Geometry check sheet. Reference: the model listing, model coordinates, mm. A direction names the side the tool comes from. Round coordinates to 2 decimals unless told otherwise and drop trailing zeros. Loops run counter-clockwise (first coordinate to the right, second up) from the corner with the lowest first, then second, coordinate; pieces in that order, holes last.
```python
from build123d import *

# Parameters (mm, degrees)
SKETCH1_W               = 30
SKETCH1_H               = 38
BOSS_EXTRUDE1_DEPTH     = 3.175
SKETCH2_W               = 30
SKETCH2_H               = 3.175
BOSS_EXTRUDE2_DEPTH     = 34.825
SKETCH3_R               = 4
CUT_EXTRUDE1_DEPTH      = 60.638751035
SKETCH4_R               = 4
CUT_EXTRUDE2_DEPTH      = 58.667679423
CROQUIS4_R              = 4
CROQUIS4_R_2            = 3.5
SALIENTE_EXTRUIR2_DEPTH = 5
CROQUIS5_W              = 3.979032683
CROQUIS5_H              = 10.100326852
CORTAR_EXTRUIR1_DEPTH   = 36
CROQUIS6_W              = 38
CROQUIS6_H              = 3.175
SALIENTE_EXTRUIR3_DEPTH = 30
CROQUIS7_W              = 3.175
CROQUIS7_H              = 34.825
SALIENTE_EXTRUIR4_DEPTH = 30
CROQUIS8_R              = 3.5
CORTAR_EXTRUIR2_DEPTH   = 30
CROQUIS9_W              = 28.045440503
CROQUIS9_H              = 19.668665091
SALIENTE_EXTRUIR5_DEPTH = 9
CROQUIS10_W             = 26.699428358
CROQUIS10_H             = 12.946692093
CORTAR_EXTRUIR3_DEPTH   = 65
CROQUIS11_R             = 3.5
CORTAR_EXTRUIR4_DEPTH   = 65


with BuildPart() as part:
    # Sketch1 → Boss-Extrude1 (new body)
    with BuildSketch(Plane.XY):
        with Locations((15, 19)):
            Rectangle(SKETCH1_W, SKETCH1_H)
    extrude(amount=BOSS_EXTRUDE1_DEPTH)

    # Sketch2 → Boss-Extrude2 (add)
    with BuildSketch(Plane(origin=(0, 0, 0), x_dir=(-1, 0, 0), z_dir=(0, 0, -1))):
        with Locations((-15, 1.5875)):
            Rectangle(SKETCH2_W, SKETCH2_H)
    extrude(amount=BOSS_EXTRUDE2_DEPTH)

    # Sketch3 → Cut-Extrude1 (cut, through all)
    with BuildSketch(Plane(origin=(0, 0, 0), x_dir=(-1, 0, 0), z_dir=(0, 0, -1))):
        with Locations((-15, 28)):
            Circle(SKETCH3_R)
    extrude(amount=-CUT_EXTRUDE1_DEPTH, mode=Mode.SUBTRACT)

    # Sketch4 → Cut-Extrude2 (cut, through all)
    with BuildSketch(Plane(origin=(0, 3.175, 0), x_dir=(1, 0, 0), z_dir=(0, 1, 0))):
        with Locations(Location((15, 24.825, 0), (0, 0, 180))):
            Circle(SKETCH4_R)
    extrude(amount=-CUT_EXTRUDE2_DEPTH, mode=Mode.SUBTRACT)

    # Croquis4 → Saliente-Extruir2 (add)
    with BuildSketch(Plane(origin=(0, 0, 0), x_dir=(-1, 0, 0), z_dir=(0, 0, -1))):
        with Locations((-15, 28)):
            Circle(CROQUIS4_R)
        with Locations((-15, 28)):
            Circle(CROQUIS4_R_2, mode=Mode.SUBTRACT)
    extrude(amount=-SALIENTE_EXTRUIR2_DEPTH)

    # Croquis5 → Cortar-Extruir1 (cut)
    with BuildSketch(Plane.ZY):
        with Locations((5.164516342, 27.585777405)):
            Rectangle(CROQUIS5_W, CROQUIS5_H)
    extrude(amount=-CORTAR_EXTRUIR1_DEPTH, mode=Mode.SUBTRACT)

    # Croquis6 → Saliente-Extruir3 (add)
    with BuildSketch(Plane.ZY):
        with Locations((-15.825, 1.5875)):
            Rectangle(CROQUIS6_W, CROQUIS6_H)
    extrude(amount=SALIENTE_EXTRUIR3_DEPTH)

    # Croquis7 → Saliente-Extruir4 (add)
    with BuildSketch(Plane.ZY):
        with Locations((1.5875, 20.5875)):
            Rectangle(CROQUIS7_W, CROQUIS7_H)
    extrude(amount=SALIENTE_EXTRUIR4_DEPTH)

    # Croquis8 → Cortar-Extruir2 (cut)
    with BuildSketch(Plane(origin=(0, 0, 0), x_dir=(-1, 0, 0), z_dir=(0, 0, -1))):
        with Locations((15, 28)):
            Circle(CROQUIS8_R)
    extrude(amount=-CORTAR_EXTRUIR2_DEPTH, mode=Mode.SUBTRACT)

    # Croquis9 → Saliente-Extruir5 (add)
    with BuildSketch(Plane(origin=(0, 3.175, 0), x_dir=(1, 0, 0), z_dir=(0, 1, 0))):
        with Locations((15.977279749, 24.990667455)):
            Rectangle(CROQUIS9_W, CROQUIS9_H)
    extrude(amount=-SALIENTE_EXTRUIR5_DEPTH)

    # Croquis10 → Cortar-Extruir3 (cut)
    with BuildSketch(Plane.ZY.offset(30)):
        with Locations((-21.475285821, -6.473346047)):
            Rectangle(CROQUIS10_W, CROQUIS10_H)
    extrude(amount=-CORTAR_EXTRUIR3_DEPTH, mode=Mode.SUBTRACT)

    # Croquis11 → Cortar-Extruir4 (cut)
    with BuildSketch(Plane(origin=(0, 3.175, 0), x_dir=(1, 0, 0), z_dir=(0, 1, 0))):
        with Locations(Location((0, 24.825, 0), (0, 0, 180))):
            Circle(CROQUIS11_R)
    extrude(amount=-CORTAR_EXTRUIR4_DEPTH, mode=Mode.SUBTRACT)


solid = part.part
```
1) Sectioned sample at B-B, the plane y = 28. Record the cut outline in (x, z) (3 decimals).
Report:
outline: (-30, 0) - (-18.5, 0) - (-18.5, 3.175) - (-30, 3.175) - close; (-11.5, 0) - (11.5, 0) - (11.5, 3.175) - (-11.5, 3.175) - close; (18.5, 0) - (30, 0) - (30, 3.175) - (18.5, 3.175) - close
2) Access from +Z, -Z, +X, -X, +Y, -Y to the whole of each face (thin tool, end or side, straight path). Record for faces 1 (the face through (0, 20, 0)), 2 (the face through (-1.615, 1.61, -27.93)).
Report:
face 1: -Z, +X, -X, +Y
face 2: +Y, -Y
3) Sectioned sample at C-C, the plane z = -26.5. Record the cut outline in (x, y) (3 decimals), then the cut area to 3 significant figures.
Report:
outline: (-30, 0) - (-3.073, 0) - (-3.073, 3.175) - (-30, 3.175) - close; (3.073, 0) - (30, 0) - (30, 3.175) - (3.073, 3.175) - close
area: 171 mm2
4) Scan lines: line 1 along Z through (x, y) = (0, 1.2) (3 decimals); line 2 along Y through (x, z) = (-26, -27) (3 decimals). Record each from-to range of solid material in increasing order.
Report:
line 1: z = -34.825 to -28.325, -21.325 to 3.175
line 2: y = 0 to 3.175
5) Sectioned sample at A-A, the plane x = 15. Record the cut outline in (y, z) (3 decimals).
Report:
outline: (0, -34.825) - (3.175, -34.825) - (3.175, 0) - (24.5, 0) - (24.5, 3.175) - (0, 3.175) - close; (31.5, 0) - (38, 0) - (38, 3.175) - (31.5, 3.175) - close
6) Gauge pin test, flat ends, axial feed: pin 1 (3 mm diameter, centred on x = -7.5, y = 24, fed in from -Z); pin 2 (2 mm diameter, centred on x = 11, z = -30.5, fed in from +Y) (3 decimals). Record the tip position at first contact, or that the pin passes through.
Report:
pin 1: stops at z = 0
pin 2: stops at y = 3.175
7) Sectioned sample at D-D, the plane x = 25.5. Record the cut outline in (y, z) (3 decimals).
Report:
outline: (0, -34.825) - (3.175, -34.825) - (3.175, 0) - (38, 0) - (38, 3.175) - (0, 3.175) - close
8) Mould release check, pull along X, two halves, no side actions. Record for faces 3 (the face through (-30, 2, -7)), 4 (the face through (-14.54, 31.47, 1.57)), 5 (the face through (30, 2, -7)), 6 (the face through (0, 0, -16)): +X half, -X half, draft (parallel to the pull), parting line (faces both ways), or undercut.
Report:
face 3: -X half
face 4: undercut
face 5: +X half
face 6: draft
